from build123d import *

# Parameters (mm, degrees)
SKETCH_1_W          = 105
SKETCH_1_H          = 52
SKETCH_1_R          = 2.025
SKETCH_1_R_2        = 1.525
SKETCH_1_W_2        = 83
SKETCH_1_H_2        = 12.5
EXTRUDE_3_DEPTH     = 4
SKETCH_3_W          = 105
SKETCH_3_H          = 12
EXTRUDE_4_DEPTH     = 4
SKETCH_6_W          = 67.640689882
SKETCH_6_H          = 62.229434692
CUT_EXTRUDE_1_DEPTH = 4
CHAMFER_1_SIZE      = 10
FILLET_2_R          = 5
SKETCH_7_W          = 20
SKETCH_7_H          = 64
SKETCH_7_R          = 1.525
EXTRUDE_5_DEPTH     = 4
SKETCH_8_W          = 12
SKETCH_8_H          = 54
CUT_EXTRUDE_2_DEPTH = 10
FILLET_3_R          = 2


with BuildPart() as part:
    # 草图1 → 凸台-拉伸3 (new body)
    with BuildSketch(Plane.XY):
        Rectangle(SKETCH_1_W, SKETCH_1_H)
        with Locations((-47.5, 4)):
            Circle(SKETCH_1_R, mode=Mode.SUBTRACT)
        with Locations((-47.5, 21)):
            Circle(SKETCH_1_R, mode=Mode.SUBTRACT)
        with Locations((-47.5, -21)):
            Circle(SKETCH_1_R, mode=Mode.SUBTRACT)
        with Locations((47.5, 21)):
            Circle(SKETCH_1_R, mode=Mode.SUBTRACT)
        with Locations((47.5, 4)):
            Circle(SKETCH_1_R, mode=Mode.SUBTRACT)
        with Locations((47.5, -21)):
            Circle(SKETCH_1_R, mode=Mode.SUBTRACT)
        with Locations((-37.5, 12.5)):
            Circle(SKETCH_1_R_2, mode=Mode.SUBTRACT)
        with Locations((37.5, 12.5)):
            Circle(SKETCH_1_R_2, mode=Mode.SUBTRACT)
        with Locations((0, 32.25)):
            Rectangle(SKETCH_1_W_2, SKETCH_1_H_2)
        with Locations((-37.5, 34.5)):
            Circle(SKETCH_1_R_2, mode=Mode.SUBTRACT)
        with Locations((37.5, 34.5)):
            Circle(SKETCH_1_R_2, mode=Mode.SUBTRACT)
    extrude(amount=EXTRUDE_3_DEPTH)

    # 草图3 → 凸台-拉伸4 (add)
    with BuildSketch(Plane.XY.offset(4)):
        with Locations((0, -32)):
            Rectangle(SKETCH_3_W, SKETCH_3_H)
        Polygon((-52.5, -26), (-52.5, 26), (-55, 26), (-55, -38), (-52.5, -38), align=None)
        Polygon((52.5, -38), (55, -38), (55, 26), (52.5, 26), (52.5, -26), align=None)
    extrude(amount=-EXTRUDE_4_DEPTH)

    # 草图6 → 切除-拉伸1 (cut)
    with BuildSketch(Plane(origin=(0, 0, 0), x_dir=(-1, 0, 0), z_dir=(0, 0, -1))):
        Rectangle(SKETCH_6_W, SKETCH_6_H)
    extrude(amount=-CUT_EXTRUDE_1_DEPTH, mode=Mode.SUBTRACT)

    # 倒角1
    chamfer_1_edges = [part.edges().sort_by_distance(p)[0] for p in [
        (-33.820344941, -31.114717346, 2),
        (33.820344941, -31.114717346, 2),
        (33.820344941, 31.114717346, 2),
        (-33.820344941, 31.114717346, 2),
    ]]
    chamfer(chamfer_1_edges, length=CHAMFER_1_SIZE)

    # 圆角2
    fillet_2_edges = [part.edges().sort_by_distance(p)[0] for p in [
        (-33.820344941, 21.114717346, 2),
        (-33.820344941, -21.114717346, 2),
        (23.820344941, -31.114717346, 2),
        (-23.820344941, -31.114717346, 2),
        (23.820344941, 31.114717346, 2),
        (-23.820344941, 31.114717346, 2),
        (33.820344941, -21.114717346, 2),
        (33.820344941, 21.114717346, 2),
    ]]
    fillet(fillet_2_edges, radius=FILLET_2_R)

    # 草图7 → 凸台-拉伸5 (add)
    with BuildSketch(Plane.XY.offset(4)):
        with Locations((-65, -6)):
            Rectangle(SKETCH_7_W, SKETCH_7_H)
        with Locations((-72, -3)):
            Circle(SKETCH_7_R, mode=Mode.SUBTRACT)
        with Locations((-72, -23)):
            Circle(SKETCH_7_R, mode=Mode.SUBTRACT)
        with Locations((65, -6)):
            Rectangle(SKETCH_7_W, SKETCH_7_H)
        with Locations((72, -23)):
            Circle(SKETCH_7_R, mode=Mode.SUBTRACT)
        with Locations((72, -3)):
            Circle(SKETCH_7_R, mode=Mode.SUBTRACT)
    extrude(amount=-EXTRUDE_5_DEPTH)

    # 草图8 → 切除-拉伸2 (cut)
    with BuildSketch(Plane.XY.offset(4)):
        with Locations((-61, -6)):
            Rectangle(SKETCH_8_W, SKETCH_8_H)
        with Locations((61, -6)):
            Rectangle(SKETCH_8_W, SKETCH_8_H)
    extrude(amount=-CUT_EXTRUDE_2_DEPTH, mode=Mode.SUBTRACT)

    # 圆角3
    fillet_3_edges = [part.edges().sort_by_distance(p)[0] for p in [
        (-75, 26, 2),
        (-75, -38, 2),
        (75, -38, 2),
        (75, 26, 2),
        (-67, -33, 2),
        (-67, 21, 2),
        (-55, 21, 2),
        (-55, -33, 2),
        (67, 21, 2),
        (67, -33, 2),
        (55, -33, 2),
        (55, 21, 2),
        (-41.5, 38.5, 2),
        (41.5, 38.5, 2),
        (41.5, 26, 2),
        (-41.5, 26, 2),
    ]]
    fillet(fillet_3_edges, radius=FILLET_3_R)


solid = part.part
Design review of the part built by this model. Coordinates are the model's own, in mm. Coordinates: 2 decimals unless noted, no trailing zeros. Loops run counter-clockwise (first coordinate to the right, second up) from the corner with the lowest first, then second, coordinate; pieces in that order, holes last.
Item 1: Draft analysis for pull direction Y (two halves, no side actions). For faces 1 (the cylindrical face through (73.4, -3.6, 2)), 2 (the flat face through (41.5, 32, 2)), state which applies: pulls with the +Y half, pulls with the -Y half, needs draft (parallel to the pull), parting line crosses it, or undercut.
Completed:
face 1: undercut
face 2: needs draft
Item 2: Clearance check with flat-ended pins moving along their axes: pin 1 (2 mm diameter, centred on x = -58, y = 21, fed in from -Z); pin 2 (1.2 mm diameter, centred on x = 59, z = 2.5, fed in from +Y). State where each tip first meets the part, or that it passes through.
Completed:
pin 1: stops at z = 0
pin 2: stops at y = 26
Item 3: Wall thickness on L1, parallel to Y at x = -47.5, z = 1.5 (3 decimals); L2, parallel to X at y = -5.5, z = 0.8; L3, parallel to Y at x = 37.5, z = 1.2 (3 decimals): over which ranges is each line inside the solid? List them lowest first.
Completed:
L1: y = -38 to -23.025, -18.975 to 1.975, 6.025 to 18.975, 23.025 to 26
L2: x = -75 to -67, -55 to -33.82, 33.82 to 55, 67 to 75
L3: y = -38 to 10.975, 14.025 to 32.975, 36.025 to 38.5
Item 4: Add section B-B (x = 37.5). Write out the cut boundary in (y, z) (3 decimals), and give its area (3 significant figures).
Completed:
outline: (-38, 0) - (10.975, 0) - (10.975, 4) - (-38, 4) - close; (14.025, 0) - (32.975, 0) - (32.975, 4) - (14.025, 4) - close; (36.025, 0) - (38.5, 0) - (38.5, 4) - (36.025, 4) - close
area: 282 mm2
Item 5: Add section C-C (x = 62.5). Write out the cut boundary in (y, z), and give its area (3 significant figures).
Completed:
outline: (-38, 0) - (-33, 0) - (-33, 4) - (-38, 4) - close; (21, 0) - (26, 0) - (26, 4) - (21, 4) - close
area: 40.0 mm2
Item 6: Add section D-D (y = -3). Write out the cut boundary in (x, z) (3 decimals), and give its area (3 significant figures).
Completed:
outline: (-75, 0) - (-73.525, 0) - (-73.525, 4) - (-75, 4) - close; (-70.475, 0) - (-67, 0) - (-67, 4) - (-70.475, 4) - close; (-55, 0) - (-33.82, 0) - (-33.82, 4) - (-55, 4) - close; (33.82, 0) - (55, 0) - (55, 4) - (33.82, 4) - close; (67, 0) - (70.475, 0) - (70.475, 4) - (67, 4) - close; (73.525, 0) - (75, 0) - (75, 4) - (73.525, 4) - close
area: 209 mm2
Item 7: Add section A-A (y = -11.5). Write out the cut boundary in (x, z), and give its area (3 significant figures).
Completed:
outline: (-75, 0) - (-67, 0) - (-67, 4) - (-75, 4) - close; (-55, 0) - (-33.82, 0) - (-33.82, 4) - (-55, 4) - close; (33.82, 0) - (55, 0) - (55, 4) - (33.82, 4) - close; (67, 0) - (75, 0) - (75, 4) - (67, 4) - close
area: 233 mm2
